Check sheet for the drawn part. Datum: minimum x, y, z corner. Units: mm. A direction names the side the tool comes from. Coordinates: 2 decimals unless noted, no trailing zeros. Order: outer loops, then holes, each group sorted by start corner. A loop starts at its lowest first (then second) coordinate and runs counter-clockwise, first axis right, second up. Notation, with made-up numbers: (70.5, -17) -> (102.5, -17) arc R26 ccw to (102.5, 17) -> close; hole circle Ø4 at (54.5, -30.75). An arc over 180 degrees is marked (long way). Answer as CSV lines item,"result".
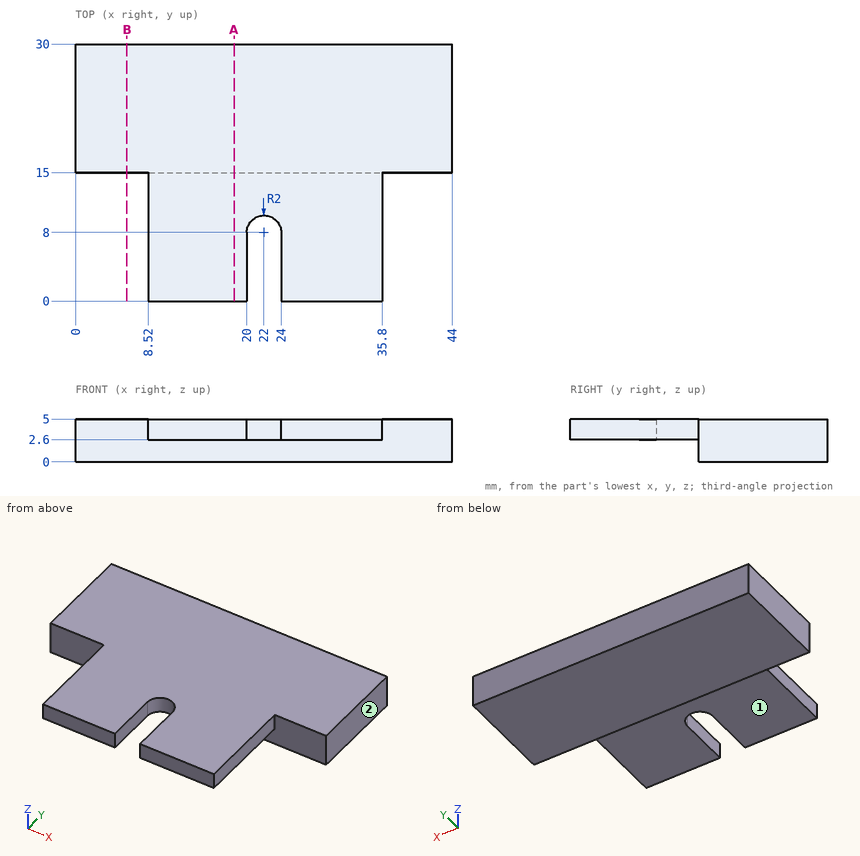
Item 1: Depth check by flat-ended pin: pin 1 Ø12 at (x, y) = (17, 4) entering from -Z; pin 2 Ø2.5 at (y, z) = (5, 4) entering from +X; pin 3 Ø1.2 at (y, z) = (3.5, 4) entering from -X. Enter the tip coordinate at first touch or a pass-through.
Answer list:
pin 1,"z = 2.6"
pin 2,"x = 35.8"
pin 3,"x = 8.52"
Item 2: Section check B-B, the plane x = 6. Record the boundary of the cut face in (y, z), plus the area to 3 significant figures.
Answer list:
outline,"(15, 0) -> (30, 0) -> (30, 5) -> (15, 5) -> close"
area,"75.0 mm2"
Item 3: Section check A-A, the plane x = 18.5. Record the boundary of the cut face in (y, z), plus the area to 3 significant figures.
Answer list:
outline,"(0, 2.6) -> (15, 2.6) -> (15, 0) -> (30, 0) -> (30, 5) -> (0, 5) -> close"
area,"111 mm2"
Item 4: Tool access check on the marked faces 1 and 2. Record the directions out of +Z, -Z, +X, -X, +Y, -Y that give a thin tool (end or side, any length) a straight path to the whole face; none if there is none.
Answer list:
face 1,"-Z, +X, -X, -Y"
face 2,"+Z, -Z, +X, +Y, -Y"
Item 5: Thickness scan on line 1 (Y direction, x = 9, z = 0.7); line 2 (Z direction, x = 9, y = 9.25); line 3 (X direction, y = 9.25, z = 4.55). Record the ranges inside material, lowest first.
Answer list:
line 1,"15 to 30"
line 2,"2.6 to 5"
line 3,"8.52 to 20.44, 23.56 to 35.8"
